Verification items for the finished model (mm, model axes). A direction names the side the tool comes from. Round coordinates to 2 decimals unless told otherwise and drop trailing zeros. Order: outer loops, then holes, each group sorted by start corner. A loop starts at its lowest first (then second) coordinate and runs counter-clockwise, first axis right, second up. Notation, with made-up numbers: M 41,4.25 L 49,4.25 A4 cw 49,8.25 Z; hole C -7.5,3.5 d11. An arc over 180 degrees is marked long. Use CSV: the item, a comma, the result in double quotes. Start each with the question number.
Q1. Gauge pin test, flat ends, axial feed: pin 1 Ø1.5 at (x, z) = (-15, -16) entering from -Y; pin 2 Ø1.5 at (x, z) = (-18, -19) entering from +Y. Record the tip position at first contact, or that the pin passes through.
Q2. Sectioned sample at A-A (z = 0). Enter the section's corners in (x, y), and give its area (3 significant figures).
Q3. Sectioned sample at B-B (x = -15.5). Enter the section's corners in (y, z).
Q4. Sectioned sample at D-D (z = 15.5). Enter the section's corners in (x, y).
Q5. Mould release check, pull along Z, two halves, no side actions. Record for faces 1 (the face through (-10, 38, 9)), 2 (the face through (0, 19, 21.15)), 3 (the face through (-20.1, 32.9, -20.2)), 4 (the face through (-15, 4.5, -15)): +Z half, -Z half, draft (parallel to the pull), parting line (faces both ways), or undercut.
Q6. Set-up check for faces 5 (the face through (-18.7, 19.4, 18.6)), 6 (the face through (15.57, 2.22, -14)), 7 (the face through (-19, 11, -19)): record each of +Z, -Z, +X, -X, +Y, -Y from which the full face is reachable in a straight line by a thin tool's end or side.
Q7. Sectioned sample at C-C (y = 26.5). Enter the section's corners in (x, z).
Q8. Scan lines: line 1 (X direction, y = 3.55, z = -15.5); line 2 (Y direction, x = 2.5, z = 16.5); line 3 (Z direction, x = 18.5, y = 25). Record each from-to range of solid material in increasing order.
```python
from build123d import *

# Parameters (mm, degrees)
BOSS_EXTRUDE1_DEPTH = 11
BOSS_EXTRUDE2_DEPTH = 17
BOSS_EXTRUDE3_DEPTH = 10
SKETCH4_R           = 11
BOSS_EXTRUDE4_DEPTH = 2
SKETCH8_R           = 1.5
CUT_EXTRUDE2_DEPTH  = 4.5


with BuildPart() as part:
    # Sketch1 → Boss-Extrude1 (new body)
    with BuildSketch(Plane(origin=(0, 0, 0), x_dir=(1, 0, 0), z_dir=(0, 1, 0))):
        Polygon((19.15, -21.15), (21.15, -19.15), (21.15, 19.15), (19.15, 21.15), (-19.15, 21.15), (-21.15, 19.15), (-21.15, -19.15), (-19.15, -21.15), align=None)
    extrude(amount=BOSS_EXTRUDE1_DEPTH)

    # Sketch2 → Boss-Extrude2 (add)
    with BuildSketch(Plane(origin=(0, 11, 0), x_dir=(1, 0, 0), z_dir=(0, 1, 0))):
        Polygon((16.15, -21.15), (21.15, -16.15), (21.15, 16.15), (16.15, 21.15), (-16.15, 21.15), (-21.15, 16.15), (-21.15, -16.15), (-16.15, -21.15), align=None)
    extrude(amount=BOSS_EXTRUDE2_DEPTH)

    # Sketch3 → Boss-Extrude3 (add)
    with BuildSketch(Plane(origin=(0, 28, 0), x_dir=(1, 0, 0), z_dir=(0, 1, 0))):
        Polygon((19.15, -21.15), (21.15, -19.15), (21.15, 19.15), (19.15, 21.15), (-19.15, 21.15), (-21.15, 19.15), (-21.15, -19.15), (-19.15, -21.15), align=None)
    extrude(amount=BOSS_EXTRUDE3_DEPTH)

    # Sketch4 → Boss-Extrude4 (add)
    with BuildSketch(Plane(origin=(0, 38, 0), x_dir=(1, 0, 0), z_dir=(0, 1, 0))):
        with Locations(Location((0, 0, 0), (0, 0, 270))):
            Circle(SKETCH4_R)
    extrude(amount=BOSS_EXTRUDE4_DEPTH)

    # Sketch8 → Cut-Extrude2 (cut)
    with BuildSketch(Plane.XZ):
        with Locations(Location((-15.5, 15.5, 0), (0, 0, 270))):
            Circle(SKETCH8_R)
        with Locations(Location((15.5, 15.5, 0), (0, 0, 270))):
            Circle(SKETCH8_R)
        with Locations(Location((15.5, -15.5, 0), (0, 0, 270))):
            Circle(SKETCH8_R)
        with Locations(Location((-15.5, -15.5, 0), (0, 0, 270))):
            Circle(SKETCH8_R)
    extrude(amount=-CUT_EXTRUDE2_DEPTH, mode=Mode.SUBTRACT)


solid = part.part
```
Verdict:
1,pin 1,"stops at y = 4.5"
1,pin 2,"stops at y = 38"
2,outline,"M -21.15,0 L 21.15,0 L 21.15,38 L 11,38 L 11,40 L -11,40 L -11,38 L -21.15,38 Z"
2,area,"1,650 mm²"
3,outline,"M 0,-21.15 L 38,-21.15 L 38,21.15 L 0,21.15 L 0,17 L 4.5,17 L 4.5,14 L 0,14 L 0,-14 L 4.5,-14 L 4.5,-17 L 0,-17 Z"
4,outline,"M -21.15,0 L -17,0 L -17,4.5 L -14,4.5 L -14,0 L 14,0 L 14,4.5 L 17,4.5 L 17,0 L 21.15,0 L 21.15,38 L -21.15,38 Z"
5,face 1,"draft"
5,face 2,"+Z half"
5,face 3,"-Z half"
5,face 4,"undercut"
6,face 5,"+Z, -X"
6,face 6,"-Y"
6,face 7,"-Z, -X"
7,outline,"M -21.15,-16.15 L -16.15,-21.15 L 16.15,-21.15 L 21.15,-16.15 L 21.15,16.15 L 16.15,21.15 L -16.15,21.15 L -21.15,16.15 Z"
8,line 1,"x = -21.15 to -17, -14 to 14, 17 to 21.15"
8,line 2,"y = 0 to 38"
8,line 3,"z = -18.8 to 18.8"
